```python
from build123d import *

# Parameters (mm, degrees)
ESBO_O1_R                 = 12.5
RESSALTO_EXTRUS_O1_DEPTH  = 20
CORTE_EXTRUS_O3_DEPTH     = 11
ESBO_O3_R                 = 6
CORTE_EXTRUS_O4_DEPTH     = 21
ESBO_O6_W                 = 12
ESBO_O6_H                 = 2
CORTE_EXTRUS_O5_DEPTH     = 10
CORTE_EXTRUS_O6_START     = -3
ESBO_O7_R                 = 3.25
CORTE_EXTRUS_O6_DEPTH     = 9.5
FURO_ROSCADO_DE_M3X0_51_D = 2.5
FILETE1_R                 = 1
ESBO_O10_R                = 1.5
CORTE_EXTRUS_O7_DEPTH     = 1
CHANFRO1_SIZE             = 0.5
CORTE_EXTRUS_O8_REACH     = 18.5
ESBO_O11_R                = 1.5
PADR_OCIRCULAR1_COUNT     = 4
CHANFRO2_SIZE             = 0.5


with BuildPart() as part:
    # Esboço1 → Ressalto-extrusão1 (new body)
    with BuildSketch(Plane.XY):
        Circle(ESBO_O1_R)
    extrude(amount=RESSALTO_EXTRUS_O1_DEPTH)

    # Esboço2 → Corte-extrusão3 (cut)
    with BuildSketch(Plane.XY.offset(20)):
        with BuildLine():
            Line((0, 0), (6.25, 10.825317547))
            ThreePointArc((6.25, 10.825317547), (12.5, 0), (6.25, -10.825317547))
            Line((6.25, -10.825317547), (0, 0))
        make_face()
    corte_extrus_o3 = extrude(amount=-CORTE_EXTRUS_O3_DEPTH, mode=Mode.SUBTRACT)

    # Esboço3 → Corte-extrusão4 (cut, through all)
    with BuildSketch(Plane(origin=(0, 0, 0), x_dir=(-1, 0, 0), z_dir=(0, 0, -1))):
        Circle(ESBO_O3_R)
    extrude(amount=-CORTE_EXTRUS_O4_DEPTH, mode=Mode.SUBTRACT)

    # Espelhar1: Corte-extrusão3 across plane
    add(corte_extrus_o3.mirror(Plane(origin=(0, 0, 0), x_dir=(0, 0, 1), z_dir=(1, 0, 0))), mode=Mode.SUBTRACT)

    # Esboço6 → Corte-extrusão5 (cut, through all)
    with BuildSketch(Plane.XY.offset(9)):
        with Locations((7, 0)):
            Rectangle(ESBO_O6_W, ESBO_O6_H)
    extrude(amount=-CORTE_EXTRUS_O5_DEPTH, mode=Mode.SUBTRACT)

    # Esboço7 → Corte-extrusão6 (cut, through all)
    with BuildSketch(Plane.XZ.offset(-1).offset(CORTE_EXTRUS_O6_START)):
        with Locations((8.459935794, 4.5)):
            Circle(ESBO_O7_R)
    extrude(amount=-CORTE_EXTRUS_O6_DEPTH, mode=Mode.SUBTRACT)

    # Furo roscado de M3x0.51 (through all)
    with Locations(Plane(origin=(0, 4, 0), x_dir=(1, 0, 0), z_dir=(0, 1, 0))):
        with Locations((8.459935794, -4.5)):
            Hole(FURO_ROSCADO_DE_M3X0_51_D / 2)

    # Filete1
    filete1_edges = [part.edges().sort_by_distance(p)[0] for p in [
        (-12.5, 0, 0),
    ]]
    fillet(filete1_edges, radius=FILETE1_R)

    # Esboço10 → Corte-extrusão7 (cut)
    with BuildSketch(Plane.XY.offset(9)):
        with Locations((6.363961031, -6.363961031)):
            Circle(ESBO_O10_R)
    corte_extrus_o7 = extrude(amount=-CORTE_EXTRUS_O7_DEPTH, mode=Mode.SUBTRACT)

    # Chanfro1
    chanfro1_edges = [part.edges().sort_by_distance(p)[0] for p in [
        (0, -12.5, 20),
        (0, 12.5, 20),
    ]]
    chamfer(chanfro1_edges, length=CHANFRO1_SIZE)

    # Esboço11 → Corte-extrusão8 (cut, up to next)
    with BuildSketch(Plane(origin=(0, 4, 0), x_dir=(1, 0, 0), z_dir=(0, 1, 0)), mode=Mode.PRIVATE) as corte_extrus_o8_sk1:
        with Locations((8.459935794, -4.5)):
            Circle(ESBO_O11_R)
    corte_extrus_o8_tool1 = extrude(corte_extrus_o8_sk1.sketch, amount=-CORTE_EXTRUS_O8_REACH, mode=Mode.PRIVATE) & part.part
    add(corte_extrus_o8_tool1.solids().sort_by_distance((8.459936, 4, 4.5))[0], mode=Mode.SUBTRACT)

    # PadrãoCircular1: Corte-extrusão7 ×4 about axis
    padr_ocircular1_axis = Axis((0, 0, 0), (0, 0, 1))
    for i in range(1, PADR_OCIRCULAR1_COUNT):
        add(corte_extrus_o7.rotate(padr_ocircular1_axis, i * 360 / PADR_OCIRCULAR1_COUNT), mode=Mode.SUBTRACT)

    # Chanfro2
    chanfro2_edges = [part.edges().sort_by_distance(p)[0] for p in [
        (-6, 0, 0),
    ]]
    chamfer(chanfro2_edges, length=CHANFRO2_SIZE)


solid = part.part
```
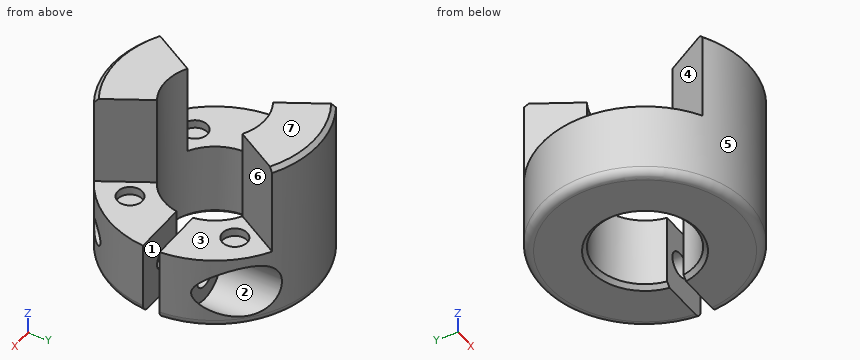
Check sheet for the modelled part. Datum: model origin and axes. Units: mm. Face numbers are marked on the shaded views. A direction names the side the tool comes from. Round coordinates to 2 decimals unless told otherwise and drop trailing zeros. Loops run counter-clockwise (first coordinate to the right, second up) from the corner with the lowest first, then second, coordinate; pieces in that order, holes last. Notation, with made-up numbers: M -17.75,43.5 L -3.75,43.5 A20 cw -3.75,47.5 Z; hole C 27,-38.75 d5. An arc over 180 degrees is marked long. Answer as a JSON object with one key per item and string values.
1. Access from +Z, -Z, +X, -X, +Y, -Y to the whole of each face (thin tool, end or side, straight path). Record for the marked faces 1, 2, 3 and 4.
Reply:
{"face 1": "+Z, -Z, +X", "face 2": "+Y", "face 3": "+Z, +X", "face 4": "+Z, -X"}
2. Mould release check, pull along Y, two halves, no side actions. Record for the marked faces 5, 6 and 7: pulls with the +Y half, pulls with the -Y half, needs draft (parallel to the pull), parting line crosses it, or undercut.
Reply:
{"face 5": "parting line crosses it", "face 6": "undercut", "face 7": "needs draft"}
3. Scan lines: line 1 (Z direction, x = -8.25, y = 2.25); line 2 (Z direction, x = 5, y = -6.75); line 3 (Y direction, x = 5.5, z = 15.5). Record each from-to range of solid material in increasing order.
Reply:
{"line 1": "z = 0 to 9", "line 2": "z = 0 to 8", "line 3": "y = -11.22 to -9.53, 9.53 to 11.22"}
4. Gauge pin test, flat ends, axial feed: P1, Ø4, axis at y = 6.5, z = 2.5, coming from the +X side; P2, Ø1.8, axis at x = -6.36, y = 6.36, coming from the +Z side; P3, Ø5, axis at y = 6.5, z = 6, coming from the -X side; P4, Ø7, axis at x = 0, y = 0, coming from the +Z side. Record the tip position at first contact, or that the pin passes through.
Reply:
{"P1": "stops at x = 11.66", "P2": "stops at z = 8", "P3": "stops at x = -11.84", "P4": "passes through"}
5. Section check C-C (z = 5). Record the boundary of the cut face in (x, y).
Reply:
{"outline": "M 5.25,4 L 5.25,11.34 A12.5 ccw long 7.31,-10.14 L 7.31,-1 L 5.92,-1 A6 cw long 5.92,1 L 7.05,1 L 7.05,4 Z; M 9.61,-8 A12.5 ccw 12.46,-1 L 9.61,-1 Z; M 9.87,1 L 12.46,1 A12.5 ccw 11.67,4.48 L 11.67,4 L 9.87,4 Z"}
6. Section check A-A (x = 0). Record the boundary of the cut face in (y, z).
Reply:
{"outline": "M -12.5,1 A1 ccw -11.5,0 L -6.5,0 L -6,0.5 L -6,20 L -12,20 L -12.5,19.5 Z; M 6,0.5 L 6.5,0 L 11.5,0 A1 ccw 12.5,1 L 12.5,19.5 L 12,20 L 6,20 Z"}
7. Section check B-B (z = 14). Record the boundary of the cut face in (x, y), plus the area to 3 significant figures.
Reply:
{"outline": "M -6.25,-10.83 A12.5 ccw 6.25,-10.83 L 3,-5.2 A6 cw -3,-5.2 Z; M -6.25,10.83 L -3,5.2 A6 cw 3,5.2 L 6.25,10.83 A12.5 ccw Z", "area": "126 mm²"}
8. Section check D-D (y = 0). Record the boundary of the cut face in (x, z).
Reply:
{"outline": "M -12.5,1 A1 ccw -11.5,0 L -6.5,0 L -6,0.5 L -6,9 L -12.5,9 Z"}
